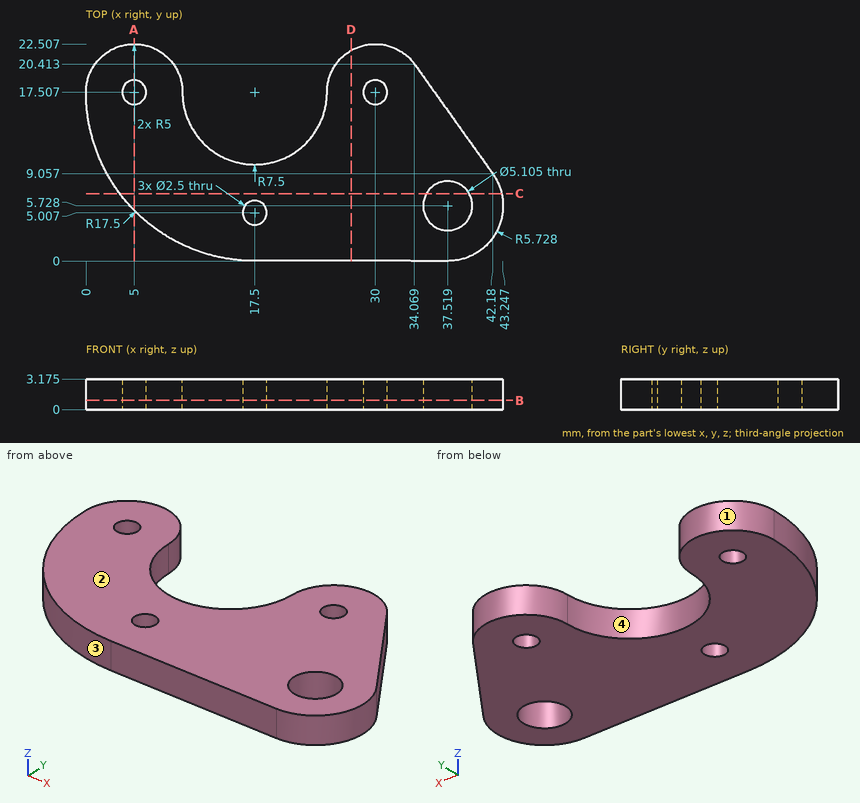
Study the drawing (mm; zero at the part's minimum x, y, z) and answer. Coordinates: 2 decimals unless noted, no trailing zeros. Order: outer loops, then holes, each group sorted by start corner. A loop starts at its lowest first (then second) coordinate and runs counter-clockwise, first axis right, second up. Notation, with made-up numbers: M -21.75,67 L 13.25,67 A24 cw 13.25,96 Z; hole C 37,78 d10. An arc over 180 degrees is marked long. Use CSV: the item, a comma, the result in double quotes.
Q1. Section C-C (y = 7) is taken. Determine the outline of the cut face in (x, z) (1 decimal), then the cut area to 3 significant figures.
Here are the results:
outline,"M 3.5,0 L 35.3,0 L 35.3,3.2 L 3.5,3.2 Z; M 39.7,0 L 43.1,0 L 43.1,3.2 L 39.7,3.2 Z"
area,"112 mm2"
Q2. Section A-A (x = 5) is taken. Determine the outline of the cut face in (y, z) (1 decimal).
Here are the results:
outline,"M 5.3,0 L 16.3,0 L 16.3,3.2 L 5.3,3.2 Z; M 18.8,0 L 22.5,0 L 22.5,3.2 L 18.8,3.2 Z"
Q3. Straight lines are drawn through the part: L1, parallel to X at y = 17.5, z = 0.85; L2, parallel to Y at x = 30, z = 2.3; L3, parallel to X at y = 19.25, z = 0.95 (1 decimal). For each, find the intervals that lie inside material, in ascending order.
Here are the results:
L1,"0 to 3.75, 6.25 to 10, 25 to 28.75, 31.25 to 36.15"
L2,"0 to 16.26, 18.76 to 22.51"
L3,"0.3 to 9.7, 25.3 to 34.9"
Q4. Section D-D (x = 27.5) is taken. Determine the outline of the cut face in (y, z) (1 decimal).
Here are the results:
outline,"M 0,0 L 21.8,0 L 21.8,3.2 L 0,3.2 Z"
Q5. Given pin 1 Ø1.5 at (x, z) = (20.5, 1.5) entering from +Y; pin 2 Ø6 at (x, y) = (21, 8.5) entering from -Z, each flat-ended and moving along its own axis, determine where each tip first touches the part or whether it passes through.
Here are the results:
pin 1,"y = 11.01"
pin 2,"z = 0"
Q6. Determine the mould class of the marked faces 1, 2, 3 and 4 for opening direction X: pulls with the +X half, pulls with the -X half, needs draft (parallel to the pull), parting line crosses it, or undercut.
Here are the results:
face 1,"undercut"
face 2,"needs draft"
face 3,"pulls with the -X half"
face 4,"undercut"
Q7. Section B-B (z = 0.95) is taken. Give the number of separate pieces and of enclosed holes in the cut face, then the cut area to 3 significant figures.
Here are the results:
separate pieces,"1"
enclosed holes,"4"
area,"605 mm2"
